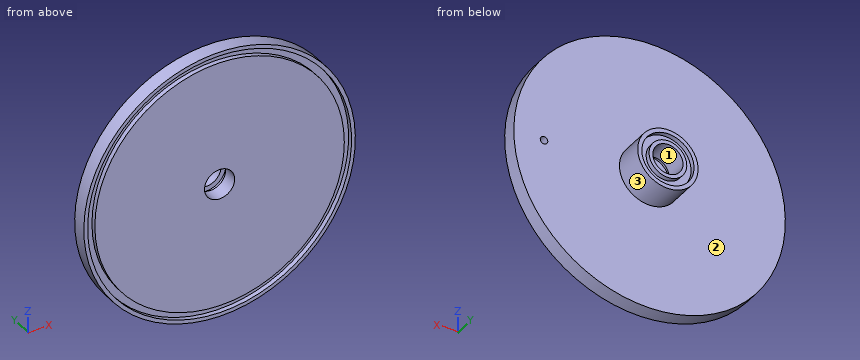
```python
from build123d import *

# Parameters (mm, degrees)
F_1_8_0_125_DIAMETER_HOLE1_D     = 3.175
F_1_8_0_125_DIAMETER_HOLE1_DEPTH = 3.175
F_1_8_0_125_DIAMETER_HOLE1_TIP   = 0.953866233


with BuildPart() as part:
    # Sketch1 → Revolve1 (revolve)
    with BuildSketch(Plane.XY, mode=Mode.PRIVATE) as revolve1_sk:
        Polygon((-6.35, 0), (-52.5145, 0), (-52.5145, 2.032), (-55.5625, 2.032), (-55.5625, 0), (-57.15, 0), (-57.15, 6.35), (-12.7, 6.35), (-12.7, 19.05), (-10.9855, 19.05), (-10.9855, 17.018), (-7.9375, 17.018), (-7.9375, 19.05), (-6.35, 19.05), (-6.35, 9.398), (-8.382, 9.398), (-8.382, 6.35), (-6.35, 6.35), align=None)
    revolve(revolve1_sk.sketch.rotate(Axis((0, 0, 0), (0, 1, 0)), 270), axis=Axis((0, 0, 0), (0, 1, 0)))

    # 1/8 (0.125) Diameter Hole1
    with Locations(Plane(origin=(0, 6.35, 0), x_dir=(1, 0, 0), z_dir=(0, 1, 0))):
        with Locations((44.45, 0)):
            Hole(F_1_8_0_125_DIAMETER_HOLE1_D / 2, depth=F_1_8_0_125_DIAMETER_HOLE1_DEPTH)
            with Locations((0, 0, -(F_1_8_0_125_DIAMETER_HOLE1_DEPTH + F_1_8_0_125_DIAMETER_HOLE1_TIP / 2))):  # 118° drill point
                Cone(0, F_1_8_0_125_DIAMETER_HOLE1_D / 2, F_1_8_0_125_DIAMETER_HOLE1_TIP, mode=Mode.SUBTRACT)


solid = part.part
```
Input: part model. Units: mm. Frame: model coordinates. Face numbers are marked on the shaded views. Give positions to 0.01 mm unless a question says otherwise; leave off trailing zeros. Order: outer loops, then holes, each group sorted by start corner. A loop starts at its lowest first (then second) coordinate and runs counter-clockwise, first axis right, second up. Notation, with made-up numbers: (69.25, 56) - (105.25, 56) arc R23 cw to (105.25, 75) - close; hole circle Ø2 at (-16.75, -38.75). An arc over 180 degrees is marked (long way). One line per item, written item: value.
1. Cut plane B-B, the plane z = -41. Output: boundary loops of the cut face in (x, y), and give its area (3 significant figures).
Determined:
outline: (-39.81, 0) - (-37.5, 0) - (-37.5, 2.03) - (-32.81, 2.03) - (-32.81, 0) - (32.81, 0) - (32.81, 2.03) - (37.5, 2.03) - (37.5, 0) - (39.81, 0) - (39.81, 6.35) - (-39.81, 6.35) - close
area: 487 mm2
2. Cut plane C-C, the plane y = 11. Output: boundary loops of the cut face in (x, z), and give its area (3 significant figures).
Determined:
outline: circle Ø25.4 at (0, 0); hole circle Ø12.7 at (0, 0)
area: 380 mm2
3. Pin query (flat end, axial travel): pin 1 Ø4 at (y, z) = (15.5, 4) entering from +X; pin 2 Ø2 at (x, y) = (-10, 7) entering from +Z; pin 3 Ø4 at (y, z) = (11, 2.5) entering from +X. Return the tip coordinate at first contact, or that it passes through.
Determined:
pin 1: x = 12.54
pin 2: z = 56.4
pin 3: x = 12.69
4. Draft query along X for the marked faces 1, 2 and 3. Return one class per face: released by +X, released by -X, zero draft, split by the parting line, or undercut.
Determined:
face 1: undercut
face 2: zero draft
face 3: split by the parting line
5. Line query: probe 1 along X at (y, z) = (0.8, 0); probe 2 along X at (y, z) = (1.75, 16); probe 3 along X at (y, z) = (7.7, 0). Output: solid intervals per line, ascending.
Determined:
probe 1: -57.15 to -55.56, -52.51 to -6.35, 6.35 to 52.51, 55.56 to 57.15
probe 2: -54.86 to -53.21, -50.02 to 50.02, 53.21 to 54.86
probe 3: -12.7 to -8.38, 8.38 to 12.7
6. Cut plane A-A, the plane x = 23.5. Output: boundary loops of the cut face in (y, z).
Determined:
outline: (0, -52.09) - (6.35, -52.09) - (6.35, 52.09) - (0, 52.09) - (0, 50.35) - (2.03, 50.35) - (2.03, 46.96) - (0, 46.96) - (0, -46.96) - (2.03, -46.96) - (2.03, -50.35) - (0, -50.35) - close
